CAD build for the part. Positions are in the model's coordinates, mm. A direction names the side the tool comes from. Round coordinates to 2 decimals unless told otherwise and drop trailing zeros. Order: outer loops, then holes, each group sorted by start corner. A loop starts at its lowest first (then second) coordinate and runs counter-clockwise, first axis right, second up. Notation, with made-up numbers: M 56,53 L 102,53 A25 cw 102,65 Z; hole C 78,-13 d11. An arc over 180 degrees is marked long. Answer as a JSON object with one key per item and string values.
```python
from build123d import *

# Parameters (mm, degrees)
SKETCH2_W               = 20
SKETCH2_H               = 50
BOSS_EXTRUDE1_DEPTH     = 44.5
SKETCH3_W               = 6.8
SKETCH3_H               = 24.75
SKETCH3_W_2             = 5
SKETCH3_H_2             = 12.5
CUT_EXTRUDE3_DEPTH      = 68.677544282
FILLET1_R               = 0.5
SKETCH7_W               = 4.6
SKETCH7_H               = 20.1
CUT_EXTRUDE4_DEPTH      = 3.25
CUT_EXTRUDE5_DEPTH      = 55.820160525
CUT_EXTRUDE5_DEPTH_BACK = 55.820160525
SKETCH8_R               = 2.6


with BuildPart() as part:
    # Sketch2 → Boss-Extrude1 (new body)
    with BuildSketch(Plane(origin=(0, 0, 0), x_dir=(1, 0, 0), z_dir=(0, 1, 0))):
        Rectangle(SKETCH2_W, SKETCH2_H)
    extrude(amount=BOSS_EXTRUDE1_DEPTH)

    # Sketch3 → Cut-Extrude3 (cut, through all)
    with BuildSketch(Plane.XY.offset(25)):
        with Locations((0, 32.125)):
            Rectangle(SKETCH3_W, SKETCH3_H)
        with Locations((0, 13.5)):
            Rectangle(SKETCH3_W_2, SKETCH3_H_2)
    extrude(amount=-CUT_EXTRUDE3_DEPTH, mode=Mode.SUBTRACT)

    # Fillet1
    fillet1_edges = [part.edges().sort_by_distance(p)[0] for p in [
        (-10, 44.5, 0),
        (-6.7, 44.5, -25),
        (6.7, 44.5, 25),
        (-6.7, 44.5, 25),
        (0, 7.25, -25),
        (-2.5, 13.5, 25),
        (2.5, 13.5, -25),
        (2.5, 19.75, 0),
        (-2.5, 13.5, -25),
        (3.4, 32.125, -25),
        (0, 7.25, 25),
        (2.5, 13.5, 25),
        (2.95, 19.75, 25),
        (-3.4, 32.125, 25),
        (-2.95, 19.75, 25),
        (-3.4, 44.5, 0),
        (3.4, 32.125, 25),
        (3.4, 44.5, 0),
        (-3.4, 32.125, -25),
        (-2.95, 19.75, -25),
        (-2.5, 19.75, 0),
        (2.95, 19.75, -25),
        (10, 44.5, 0),
        (0, 0, 25),
        (-10, 0, 0),
        (0, 0, -25),
        (10, 0, 0),
        (10, 22.25, 25),
        (-10, 22.25, 25),
        (-10, 22.25, -25),
        (10, 22.25, -25),
        (6.7, 44.5, -25),
    ]]
    fillet(fillet1_edges, radius=FILLET1_R)

    # Sketch7 → Cut-Extrude4 (cut)
    with BuildSketch(Plane.ZY.offset(10)):
        with Locations((16.3, 13.53)):
            Rectangle(SKETCH7_W, SKETCH7_H)
    extrude(amount=-CUT_EXTRUDE4_DEPTH, mode=Mode.SUBTRACT)

    # Sketch8 → Cut-Extrude5 (cut, two sides: drawn at the far end of the back side and taken through both)
    with BuildSketch(Plane.ZY.offset(10).offset(-CUT_EXTRUDE5_DEPTH_BACK)):
        with Locations((-13, 32.41)):
            Circle(SKETCH8_R)
        with Locations((12.4, 32.41)):
            Circle(SKETCH8_R)
    extrude(amount=CUT_EXTRUDE5_DEPTH + CUT_EXTRUDE5_DEPTH_BACK, mode=Mode.SUBTRACT)


solid = part.part
```
Item 1: Saw through at D-D on z = 4. List the corners of the cut face in (x, y).
Worked answers:
{"outline": "M -10,0.5 A0.5 ccw -9.5,0 L 9.5,0 A0.5 ccw 10,0.5 L 10,44 A0.5 ccw 9.5,44.5 L 3.9,44.5 A0.5 ccw 3.4,44 L 3.4,19.75 L 3,19.75 A0.5 ccw 2.5,19.25 L 2.5,7.25 L -2.5,7.25 L -2.5,19.25 A0.5 ccw -3,19.75 L -3.4,19.75 L -3.4,44 A0.5 ccw -3.9,44.5 L -9.5,44.5 A0.5 ccw -10,44 Z"}
Item 2: Wall check: line 1 along Z through (x, y) = (5.25, 32.41); line 2 along X through (y, z) = (27, 6.5); line 3 along Y through (x, z) = (5, 12.4). Give the ranges that are in metal, low to high. Write a range as [from, to].
Worked answers:
{"line 1": "z = [-25, -15.6], [-10.4, 9.8], [15, 25]", "line 2": "x = [-10, -3.4], [3.4, 10]", "line 3": "y = [0, 29.81], [35.01, 44.5]"}
Item 3: Saw through at C-C on y = 32.41. State how many separate pieces and enclosed holes the cut face has, and give its area (3 significant figures).
Worked answers:
{"separate pieces": "6", "enclosed holes": "0", "area": "522 mm2"}
Item 4: Drop flat-ended pins along their axis: pin 1 Ø6 at (y, z) = (31.5, 14.5) entering from +X; pin 2 Ø5.5 at (x, z) = (0, 10.5) entering from +Y. Give the stop position or say it passes through.
Worked answers:
{"pin 1": "stops at x = 10", "pin 2": "stops at y = 19.68"}
Item 5: Saw through at A-A on z = -13. List the corners of the cut face in (x, y).
Worked answers:
{"outline": "M -10,0.5 A0.5 ccw -9.5,0 L 9.5,0 A0.5 ccw 10,0.5 L 10,29.81 L 3.4,29.81 L 3.4,19.75 L 3,19.75 A0.5 ccw 2.5,19.25 L 2.5,7.25 L -2.5,7.25 L -2.5,19.25 A0.5 ccw -3,19.75 L -3.4,19.75 L -3.4,29.81 L -10,29.81 Z; M -10,35.01 L -3.4,35.01 L -3.4,44 A0.5 ccw -3.9,44.5 L -9.5,44.5 A0.5 ccw -10,44 Z; M 3.4,35.01 L 10,35.01 L 10,44 A0.5 ccw 9.5,44.5 L 3.9,44.5 A0.5 ccw 3.4,44 Z"}
Item 6: Saw through at B-B on y = 38. List the corners of the cut face in (x, z), and give its area (3 significant figures).
Worked answers:
{"outline": "M -10,-24.5 A0.5 ccw -9.5,-25 L -3.9,-25 A0.5 ccw -3.4,-24.5 L -3.4,24.5 A0.5 ccw -3.9,25 L -9.5,25 A0.5 ccw -10,24.5 Z; M 3.4,-24.5 A0.5 ccw 3.9,-25 L 9.5,-25 A0.5 ccw 10,-24.5 L 10,24.5 A0.5 ccw 9.5,25 L 3.9,25 A0.5 ccw 3.4,24.5 Z", "area": "660 mm2"}
Item 7: Two-plate mould, pull along Z, no slides. Class faces 4 (the cylindrical face through (6.75, 31.41, 14.8)), 5 (the flat face through (10, 22, 0)), 6 (the flat face through (4.1, 21.9, -25)): released by +Z, released by -Z, zero draft, split by the parting line, or undercut.
Worked answers:
{"face 4": "undercut", "face 5": "zero draft", "face 6": "released by -Z"}
Item 8: 3-axis set-ups, long thin cutter, end or side, ignore diameter. For faces 1 (the flat face through (-6.75, 14, 16)), 2 (the flat face through (2.5, 13, 0)), 3 (the cylindrical face through (-6.65, 31.41, 14.8)): which of +Z, -Z, +X, -X, +Y, -Y reach the whole face in a straight line?
Worked answers:
{"face 1": "-X", "face 2": "+Z, -Z, +Y", "face 3": "+X, -X"}
